Design review of the part built by this model. Coordinates are the model's own, in mm. A direction names the side the tool comes from. Round coordinates to 2 decimals unless told otherwise and drop trailing zeros. Write each loop counter-clockwise with the first axis right and the second up, starting at its lowest first coordinate (ties: lowest second). Pieces come first, ordered by that corner, then holes. Notation, with made-up numbers: M 59.5,89 L 110.5,89 A26 cw 110.5,120 Z; hole C -20,-40 d11. An arc over 180 degrees is marked long. One line per question, with ' | ' between items. Start each with the question number.
Item 1: Add section A-A, the plane y = 0. State the section outline as (x, z) points, and give its area (3 significant figures).
Item 2: Add section B-B, the plane z = 2.1. State the section outline as (x, y) points.
Item 3: Insertion check: pin 1 Ø1 at (y, z) = (-2.5, 1) entering from -X. The pin has a flat end and moves straight along its axis. Give the tip position at first contact, or say it passes through.
Item 4: Draft analysis for pull direction Y (two halves, no side actions). For faces 1 (the face through (1, 7, 0)), 2 (the face through (-5, -6.2, 1)), 3 (the face through (-16.4, 0, 1)), 4 (the face through (85, 0, 1)), state which applies: released by +Y, released by -Y, zero draft, split by the parting line, or undercut.
Item 5: For L1, parallel to Y at x = 1, z = 0.5; L2, parallel to Y at x = -75, z = 1.15; L3, parallel to X at y = 1.5, z = 1.9, list the stretches that pass through material, from the lowest coordinate up.
Item 6: Machinability: for faces 5 (the face through (1, -10, 1)), 6 (the face through (6.2, 0, 1)), which of the approach directions +Z, -Z, +X, -X, +Y, -Y give a long, thin tool a straight path to every point of the face, cutting with its end or side? Answer none if there is none.
Item 7: Add section C-C, the plane y = 8.5. State the section outline as (x, z) points, and give its area (3 significant figures).
```python
from build123d import *

# Parameters (mm, degrees)
SKETCH1_R           = 3
SKETCH1_W           = 22.6
SKETCH1_H           = 12.4
BOSS_EXTRUDE1_DEPTH = 3


with BuildPart() as part:
    # Sketch1 → Boss-Extrude1 (new body)
    with BuildSketch(Plane.XY):
        with BuildLine():
            Line((75, -10), (-75, -10))
            ThreePointArc((-75, -10), (-85, 0), (-75, 10))
            Line((-75, 10), (75, 10))
            ThreePointArc((75, 10), (85, 0), (75, -10))
        make_face()
        with Locations((75, 0)):
            Circle(SKETCH1_R, mode=Mode.SUBTRACT)
        with Locations((-75, 0)):
            Circle(SKETCH1_R, mode=Mode.SUBTRACT)
        with Locations((-5.1, 0)):
            Rectangle(SKETCH1_W, SKETCH1_H, mode=Mode.SUBTRACT)
    extrude(amount=BOSS_EXTRUDE1_DEPTH)


solid = part.part
```
Computed values:
1) outline: M -85,0 L -78,0 L -78,3 L -85,3 Z; M -72,0 L -16.4,0 L -16.4,3 L -72,3 Z; M 6.2,0 L 72,0 L 72,3 L 6.2,3 Z; M 78,0 L 85,0 L 85,3 L 78,3 Z | area: 406 mm^2
2) outline: M -75,-10 L 75,-10 A10 ccw 75,10 L -75,10 A10 ccw Z; hole C -75,0 d6; hole M -16.4,-6.2 L 6.2,-6.2 L 6.2,6.2 L -16.4,6.2 Z; hole C 75,0 d6
3) pin 1: stops at x = -84.8
4) face 1: zero draft | face 2: undercut | face 3: undercut | face 4: split by the parting line
5) L1: y = -10 to -6.2, 6.2 to 10 | L2: y = -10 to -3, 3 to 10 | L3: x = -84.89 to -77.6, -72.4 to -16.4, 6.2 to 72.4, 77.6 to 84.89
6) face 5: +Z, -Z, +X, -X, -Y | face 6: +Z, -Z
7) outline: M -80.27,0 L 80.27,0 L 80.27,3 L -80.27,3 Z | area: 482 mm^2
